Could you check a few things on this model? Use its own coordinates, in mm. A direction names the side the tool comes from. Give positions to 0.01 mm unless a question says otherwise; leave off trailing zeros. Order: outer loops, then holes, each group sorted by start corner. A loop starts at its lowest first (then second) coordinate and runs counter-clockwise, first axis right, second up. Notation, with made-up numbers: (82.5, 88) -> (95.5, 88) arc R23 cw to (95.5, 111) -> close; hole circle Ø7 at (59, 47.25). An arc over 180 degrees is marked (long way). Write each question's results on one line, items separated by ' | '.
Autodesk Inventor part; units mm, degrees
ref_plane "YZ Plane" through (0, 0, 0) normal (1, 0, 0) x (0, 1, 0)
ref_plane "XZ Plane" through (0, 0, 0) normal (0, 1, 0) x (-1, 0, 0)
ref_plane "XY Plane" through (0, 0, 0) normal (0, 0, 1) x (1, 0, 0)
sketch "Esquisse2" plane through (0, 0, 0) normal (0, 1, 0) x (-1, 0, 0)
  circle A0 centre (0, 0) radius 37.5
  line L0 (45, 37.5) -> (45, -37.5)
  line L1 (45, -37.5) -> (45, -40.5)
  line L2 (45, -40.5) -> (0, -40.5)
  line L3 (0, -40.5) -> (0, -37.5)
  line L4 (0, 37.5) -> (0, 40.5)
  line L5 (0, 40.5) -> (45, 40.5)
  line L6 (45, 40.5) -> (45, 37.5)
  point P0 (22.5, 40.5)
  dimension "d0" = 75
  dimension "d4" = 81
  dimension "d13" = 45
  dimension "d14" = 45
extrude "Extrusion1" add sketch "Esquisse2" along normal blind 50 contours A0 L4 L5 L6 L0 L1 L2 L3
sketch "Esquisse3" plane through (-45, 0, -40.5) normal (-1, 0, 0) x (0, 0, 1)
  line L0 (61, 15) -> (20, 15)
  line L1 (20, 15) -> (20, 35)
  line L2 (20, 35) -> (61, 35)
  line L3 (61, 35) -> (61, 15)
  line L4 (81, 0) -> (81, 50)
  line L5 (0, 0) -> (0, 50)
  line L6 (0, 0) -> (81, 0)
  line L7 (0, 50) -> (81, 50)
  point P0 (40.5, 0)
  point P1 (61, 25)
  dimension "d7" = 20
  dimension "d8" = 20
  dimension "d9" = 15
  dimension "d10" = 15
extrude "Extrusion2" cut sketch "Esquisse3" against normal blind 50 contours L0 L1 L2 L3
sketch "Esquisse4" plane through (-45, 0, -40.5) normal (-1, 0, 0) x (0, 0, 1)
  line L0 (61, 15) -> (20, 15)
  line L1 (20, 15) -> (40.5, 15)
  line L2 (40.5, 15) -> (40.5, 9)
  line L3 (40.5, 9) -> (20, 9)
  line L4 (20, 9) -> (20, 15)
  point P0 (40.5, 0)
extrude "Extrusion3" add sketch "Esquisse4" along normal blind 20
sketch "Esquisse5" plane through (-45, 9, -20.5) normal (0, -1, 0) x (1, 0, 0)
  circle A0 centre (-10, 10) radius 5
  point P0 (45, 20.5)
  dimension "d17" = 10
extrude "Extrusion4" cut sketch "Esquisse5" against normal blind 20
properties part number "corps_pince_aimant"
Q1. Suppose I cut it at D-D on z = -10.5. Please give me the cut outline in (x, y).
Here are the results:
outline: (-65, 9) -> (-60, 9) -> (-60, 15) -> (-65, 15) -> close; (-50, 9) -> (-45, 9) -> (-45, 0) -> (-36, 0) -> (-36, 15) -> (-50, 15) -> close; (-45, 35) -> (-36, 35) -> (-36, 50) -> (-45, 50) -> close
Q2. For faces 1 (the flat face through (-52.6, 9, -5.6)), 2 (the flat face through (-55, 12, 0)), 3 (the flat face through (-40, 35, 0)), which set-ups out of +Z, -Z, +X, -X, +Y, -Y let a thin tool reach every point of the face, with its end or its side?
Here are the results:
face 1: +Z, -Z, -X, -Y | face 2: +Z, -X, +Y, -Y | face 3: +X, -X
Q3. Suppose I cut it at B-B on y = 13. Please give me the cut outline in (x, z), and give its area (3 significant figures).
Here are the results:
outline: (-65, -20.5) -> (-45, -20.5) -> (-45, -40.5) -> (0, -40.5) -> (0, -37.5) arc R37.5 cw to (0, 37.5) -> (0, 40.5) -> (-45, 40.5) -> (-45, 0) -> (-65, 0) -> close; hole circle Ø10 at (-55, -10.5) | area: 1,770 mm²
Q4. I'm going to push flat-ended pins straight in: pin 1 Ø6 at (x, z) = (-56.5, -5.5) entering from -Y; pin 2 Ø5 at (y, z) = (37.5, -29.5) entering from -X; pin 3 Ø11.5 at (x, z) = (-55, -10.5) entering from +Y; pin 4 Ø6 at (y, z) = (12, -21.5) entering from -X. Where does each tip first touch, or does it pass through?
Here are the results:
pin 1: stops at y = 9 | pin 2: stops at x = -45 | pin 3: stops at y = 15 | pin 4: stops at x = -65
Q5. Suppose I cut it at C-C on x = -40. Please give me the cut outline in (y, z).
Here are the results:
outline: (0, -40.5) -> (50, -40.5) -> (50, 40.5) -> (0, 40.5) -> close; hole (15, -20.5) -> (35, -20.5) -> (35, 20.5) -> (15, 20.5) -> close
Q6. I need wall thicknesses on line 1 along Z through (x, y) = (-55, 12.3); line 2 along Z through (x, y) = (-35, 23.5); line 3 along Y through (x, z) = (-36.5, -16). Which ranges of each line are inside material? Lowest first, please.
Here are the results:
line 1: z = -20.5 to -15.5, -5.5 to 0 | line 2: z = -40.5 to -20.5, 20.5 to 40.5 | line 3: y = 0 to 15, 35 to 50
Q7. Suppose I cut it at A-A on y = 33.5. Please give me the cut outline in (x, z), and give its area (3 significant figures).
Here are the results:
outline: (-45, -40.5) -> (0, -40.5) -> (0, -37.5) arc R37.5 cw to (-31.4, -20.5) -> (-45, -20.5) -> close; (-45, 20.5) -> (-31.4, 20.5) arc R37.5 cw to (0, 37.5) -> (0, 40.5) -> (-45, 40.5) -> close | area: 1,050 mm²
Q8. Thinking about a two-plate mould opening in Y: for faces 4 (the flat face through (-37, 0, 10)), 5 (the flat face through (-55, 12, -20.5)), 6 (the flat face through (-44, 15, -4)), which applies, +Y half, -Y half, draft (parallel to the pull), parting line (faces both ways), or undercut?
Here are the results:
face 4: -Y half | face 5: draft | face 6: undercut
